Design review of the part built by this model. Coordinates are the model's own, in mm. A direction names the side the tool comes from. Coordinates: 2 decimals unless noted, no trailing zeros. Loops run counter-clockwise (first coordinate to the right, second up) from the corner with the lowest first, then second, coordinate; pieces in that order, holes last. Notation, with made-up numbers: (-22.75, -34) - (8.25, -34) arc R4 ccw to (8.25, -29) - close; hole circle Ø8 at (57.25, 13.5). An arc over 180 degrees is marked (long way). One line per question, with ' | ' between items.
from build123d import *

# Parameters (mm, degrees)
SKETCH1_W           = 39
SKETCH1_H           = 14.65
BOSS_EXTRUDE1_DEPTH = 9.5
SKETCH2_W           = 18
SKETCH2_H           = 14.65
BOSS_EXTRUDE2_DEPTH = 15.5
SKETCH3_R           = 1.5
CUT_EXTRUDE1_DEPTH  = 15.5


with BuildPart() as part:
    # Sketch1 → Boss-Extrude1 (new body)
    with BuildSketch(Plane.XY):
        with Locations((19.5, 7.325)):
            Rectangle(SKETCH1_W, SKETCH1_H)
    extrude(amount=BOSS_EXTRUDE1_DEPTH)

    # Sketch2 → Boss-Extrude2 (add)
    with BuildSketch(Plane.XY.offset(9.5)):
        with Locations((19.5, 7.325)):
            Rectangle(SKETCH2_W, SKETCH2_H)
    extrude(amount=BOSS_EXTRUDE2_DEPTH)

    # Sketch3 → Cut-Extrude1 (cut)
    with BuildSketch(Plane(origin=(0, 0, 0), x_dir=(-1, 0, 0), z_dir=(0, 0, -1))):
        with Locations((-32.7, 7.325)):
            Circle(SKETCH3_R)
        with Locations((-6.3, 7.325)):
            Circle(SKETCH3_R)
    extrude(amount=-CUT_EXTRUDE1_DEPTH, mode=Mode.SUBTRACT)


solid = part.part
Q1. Draft analysis for pull direction X (two halves, no side actions). For faces 4 (the flat face through (4, 7, 9.5)), 5 (the cylindrical face through (7, 6, 5)), 6 (the flat face through (0, 7, 5)), state which applies: +X half, -X half, draft (parallel to the pull), parting line (faces both ways), or undercut.
Returned:
face 4: draft | face 5: undercut | face 6: -X half
Q2. Tool access review of faces 1 (the flat face through (19, 0, 10)), 2 (the flat face through (35, 7, 9.5)), 3 (the flat face through (10.5, 7, 17)): name each direction out of +Z, -Z, +X, -X, +Y, -Y from which nothing blocks a thin tool from reaching the whole face with its end or side.
Returned:
face 1: +Z, -Z, +X, -X, -Y | face 2: +Z, +X, +Y, -Y | face 3: +Z, -X, +Y, -Y
Q3. Take a section at B-B (y = 11.25). Give the boundary of the cut face in (x, z).
Returned:
outline: (0, 0) - (39, 0) - (39, 9.5) - (28.5, 9.5) - (28.5, 25) - (10.5, 25) - (10.5, 9.5) - (0, 9.5) - close
Q4. Take a section at C-C (z = 6.5). Give the boundary of the cut face in (x, y) (3 decimals).
Returned:
outline: (0, 0) - (39, 0) - (39, 14.65) - (0, 14.65) - close; hole circle Ø3 at (6.3, 7.325); hole circle Ø3 at (32.7, 7.325)
Q5. Take a section at D-D (x = 4). Give the boundary of the cut face in (y, z), plus the area to 3 significant figures.
Returned:
outline: (0, 0) - (14.65, 0) - (14.65, 9.5) - (0, 9.5) - close | area: 139 mm²
Q6. To check wall thickness, follow line 1 along Y through (x, z) = (6.3, 3.75) (3 decimals); line 2 along X through (y, z) = (7.5, 10.75); line 3 along Z through (x, y) = (31, 13). State the ranges of each line that lie inside material, in increasing order.
Returned:
line 1: y = 0 to 5.825, 8.825 to 14.65 | line 2: x = 10.5 to 28.5 | line 3: z = 0 to 9.5
Q7. For pin 1 (2.5 mm diameter, centred on x = 6.3, y = 7.325, fed in from +Z); pin 2 (3 mm diameter, centred on x = 36, y = 5, fed in from +Z); pin 3 (1.5 mm diameter, centred on y = 10, z = 18.5, fed in from +X), all flat-tipped, find the tip position at first contact; note any pin that passes through.
Returned:
pin 1: passes through | pin 2: stops at z = 9.5 | pin 3: stops at x = 28.5
Q8. Take a section at A-A (x = 32.7). Give the boundary of the cut face in (y, z) (3 decimals), plus the area to 3 significant figures.
Returned:
outline: (0, 0) - (5.825, 0) - (5.825, 9.5) - (0, 9.5) - close; (8.825, 0) - (14.65, 0) - (14.65, 9.5) - (8.825, 9.5) - close | area: 111 mm²
